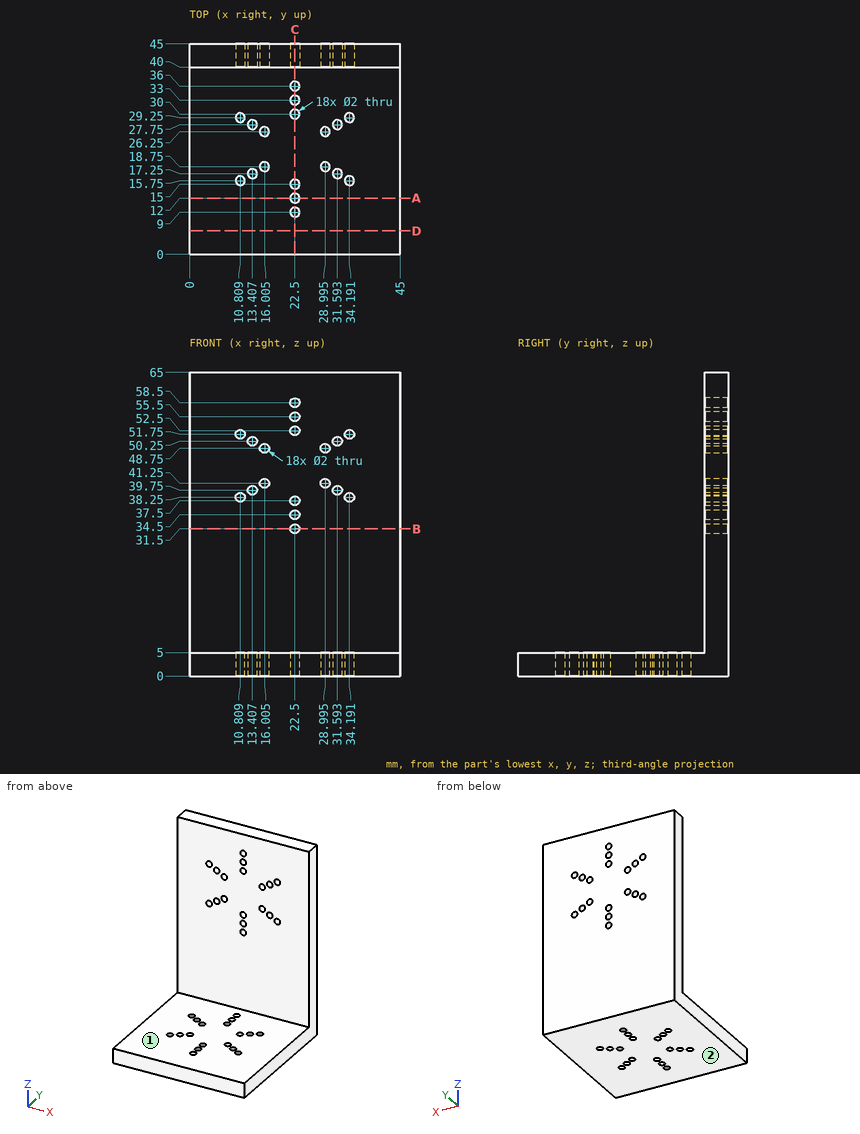
The drawing under review shows one solid part. Ordinate dimensions are in mm from its lowest x, y, z. A direction names the side the tool comes from. Give positions to 0.01 mm unless a question says otherwise; leave off trailing zeros. Order: outer loops, then holes, each group sorted by start corner. A loop starts at its lowest first (then second) coordinate and runs counter-clockwise, first axis right, second up. Notation, with made-up numbers: (1, 41.5) -> (10, 41.5) arc R21 ccw to (10, 56.5) -> close; hole circle Ø1 at (11.25, 64.5). An arc over 180 degrees is marked (long way). Write item = value, one per line.
1) For the marked faces 1 and 2, list the 3-axis set-ups (+Z, -Z, +X, -X, +Y, -Y) from which the entire face can be reached by the end or side of a thin tool; tool diameter is ignored.
Findings:
face_1 = +Z, +X, -X, -Y
face_2 = -Z, +X, -X, +Y, -Y
2) We need section B-B, the plane z = 31.5. Give the boundary of the cut face in (x, y), and give its area (3 significant figures).
Findings:
outline = (0, 40) -> (21.5, 40) -> (21.5, 45) -> (0, 45) -> close; (23.5, 40) -> (45, 40) -> (45, 45) -> (23.5, 45) -> close
area = 215 mm^2
3) We need section A-A, the plane y = 12. Give the boundary of the cut face in (x, z).
Findings:
outline = (0, 0) -> (21.5, 0) -> (21.5, 5) -> (0, 5) -> close; (23.5, 0) -> (45, 0) -> (45, 5) -> (23.5, 5) -> close
4) Insertion check: pin 1 (5 mm diameter, centred on x = 6, y = 6, fed in from +Z); pin 2 (1.2 mm diameter, centred on x = 31.59, z = 39.75, fed in from +Y); pin 3 (1 mm diameter, centred on x = 9.5, z = 42, fed in from -Y). Each pin has a flat end and moves straight along its axis. Give the tip position at first contact, or say it passes through.
Findings:
pin_1 = 5
pin_2 = through
pin_3 = 40
5) To check wall thickness, follow L1, parallel to X at y = 41.65, z = 48.75 (1 decimal); L2, parallel to X at y = 43, z = 52 (1 decimal); L3, parallel to Y at x = 26, z = 43. State the ranges of each line that lie inside material, in increasing order. Write a range as from..to.
Findings:
L1 = 0..15, 17..28, 30..45
L2 = 0..9.8, 11.8..21.6, 23.4..33.2, 35.2..45
L3 = 40..45
6) We need section C-C, the plane x = 22.5. Count the separate pieces of the cut face and the enclosed holes in it, and give its area (3 significant figures).
Findings:
separate_pieces = 13
enclosed_holes = 0
area = 405 mm^2
7) We need section D-D, the plane y = 5. Give the boundary of the cut face in (x, z), and give its area (3 significant figures).
Findings:
outline = (0, 0) -> (45, 0) -> (45, 5) -> (0, 5) -> close
area = 225 mm^2
